```python
from build123d import *

# Parameters (mm, degrees)
HOLE_WIZARD_M41_D     = 4.8
HOLE_WIZARD_M41_DEPTH = 16
HOLE_WIZARD_M41_TIP   = 1.442065486
CUT_EXTRUDE_1_DEPTH   = 2.2


with BuildPart() as part:
    # Эскиз1 → Повернуть1 (revolve)
    with BuildSketch(Plane(origin=(0, 0, 0), x_dir=(0, 0, -1), z_dir=(1, 0, 0))):
        Polygon((0, 0), (-23, 0), (-23, -4.5), (-22, -5.5), (0, -5.5), align=None)
    revolve(axis=Axis((0, 0, 28.650369954), (0, 0, -1)))

    # Отверстие с зазором M41
    with Locations(Plane(origin=(0, 0, 23), x_dir=(0, 1, 0), z_dir=(0, 0, 1))):
        with Locations((0, 0)):
            Hole(HOLE_WIZARD_M41_D / 2, depth=HOLE_WIZARD_M41_DEPTH)
            with Locations((0, 0, -(HOLE_WIZARD_M41_DEPTH + HOLE_WIZARD_M41_TIP / 2))):  # 118° drill point
                Cone(0, HOLE_WIZARD_M41_D / 2, HOLE_WIZARD_M41_TIP, mode=Mode.SUBTRACT)

    # Эскиз4 → Вырез-Вытянуть1 (cut)
    with BuildSketch(Plane(origin=(0, 5.5, 0), x_dir=(1, 0, 0), z_dir=(0, 1, 0))):
        Polygon((0, -19), (2, -19), (2, -3), (-2, -3), (-2, -19), align=None)
    extrude(amount=-CUT_EXTRUDE_1_DEPTH, mode=Mode.SUBTRACT)


solid = part.part
```
Design review of the part built by this model. Coordinates are the model's own, in mm. A direction names the side the tool comes from. Give positions to 0.01 mm unless a question says otherwise; leave off trailing zeros. Loops run counter-clockwise (first coordinate to the right, second up) from the corner with the lowest first, then second, coordinate; pieces in that order, holes last. Notation, with made-up numbers: (89.5, -22.75) -> (117.5, -22.75) arc R19 cw to (117.5, -5.75) -> close; hole circle Ø8 at (-26, 45). An arc over 180 degrees is marked (long way). One line per item, written item: value.
Q1. We need section B-B on z = 3.75. Give the boundary of the cut face in (x, y).
Numbers:
outline: (-2, 3.3) -> (-2, 5.12) arc R5.5 ccw (long way) to (2, 5.12) -> (2, 3.3) -> close
Q2. Draft analysis for pull direction Z (two halves, no side actions). For faces 1 (the flat face through (0, 0, 0)), 2 (the flat face through (0, 4, 19)), 3 (the flat face through (2, 2, 23)), state which applies: pulls with the +Z half, pulls with the -Z half, needs draft (parallel to the pull), parting line crosses it, or undercut.
Numbers:
face 1: pulls with the -Z half
face 2: undercut
face 3: pulls with the +Z half
Q3. For pin 1 Ø5 at (x, y) = (0, -1) entering from -Z; pin 2 Ø1.5 at (y, z) = (4, 9.5) entering from -X; pin 3 Ø4 at (x, z) = (-3, 16) entering from -Y; pin 4 Ø5 at (y, z) = (3, 5) entering from -X, all flat-tipped, find the tip position at first contact; note any pin that passes through.
Numbers:
pin 1: stops at z = 0
pin 2: stops at x = -4.44
pin 3: stops at y = -5.41
pin 4: stops at x = -5.48
Q4. For L1, parallel to X at y = 0, z = 14; L2, parallel to X at y = 4, z = 7; L3, parallel to X at y = 0.25, z = 3.75, list the stretches that pass through material, from the lowest coordinate up.
Numbers:
L1: x = -5.5 to -2.4, 2.4 to 5.5
L2: x = -3.77 to -2, 2 to 3.77
L3: x = -5.49 to 5.49
Q5. We need section A-A on z = 14. Give the boundary of the cut face in (x, y), and give its area (3 significant figures).
Numbers:
outline: (-2, 3.3) -> (-2, 5.12) arc R5.5 ccw (long way) to (2, 5.12) -> (2, 3.3) -> close; hole circle Ø4.8 at (0, 0)
area: 68.6 mm^2
Q6. Machinability: for faces 4 (the cylindrical face through (-2.024, -1.29, 14.888)), 5 (the cylindrical face through (2.11, -5.08, 10.85)), 6 (the flat face through (0, 3.3, 11)), which of the approach directions +Z, -Z, +X, -X, +Y, -Y give a long, thin tool a straight path to every point of the face, cutting with its end or side? Answer none if there is none.
Numbers:
face 4: +Z
face 5: +Z, -Z
face 6: +Y
